from build123d import *

# Parameters (mm, degrees)
SKETCH1_W                           = 139.7
SKETCH1_H                           = 127
BOSS_EXTRUDE1_DEPTH                 = 12
F_8_CLEARANCE_HOLE1_D               = 4.9149
SKETCH2_R                           = 43.18
SKETCH2_R_2                         = 4.7625
CUT_EXTRUDE1_DEPTH                  = 1.27
SKETCH2_4_R                         = 4.7625
CUT_EXTRUDE2_DEPTH                  = 96.159195562
TAP_DRILL_FOR_10_24_TAP1_AT_2_COUNT = 2
TAP_DRILL_FOR_10_24_TAP1_AT_2_PITCH = 50.8
TAP_DRILL_FOR_10_24_TAP1_AT_3_COUNT = 2
TAP_DRILL_FOR_10_24_TAP1_AT_3_PITCH = 101.6
SKETCH8_R                           = 5.715
CUT_EXTRUDE3_DEPTH                  = 0.889


with BuildPart() as part:
    # Sketch1 → Boss-Extrude1 (new body)
    with BuildSketch(Plane(origin=(0, 0, 0), x_dir=(0, 0, -1), z_dir=(1, 0, 0))):
        Rectangle(SKETCH1_W, SKETCH1_H)
    extrude(amount=BOSS_EXTRUDE1_DEPTH)

    # #8 Clearance Hole1 (through all)
    with Locations(Plane.ZY):
        with Locations((-32.786915098, 34.756915098), (32.786915098, 34.756915098), (32.786915098, -30.816915098), (-32.786915098, -30.816915098)):
            Hole(F_8_CLEARANCE_HOLE1_D / 2)

    # Sketch2 → Cut-Extrude1 (cut)
    with BuildSketch(Plane.ZY):
        with Locations((0, 1.97)):
            Circle(SKETCH2_R)
        with Locations((0, 1.97)):
            Circle(SKETCH2_R_2, mode=Mode.SUBTRACT)
    extrude(amount=-CUT_EXTRUDE1_DEPTH, mode=Mode.SUBTRACT)

    # Sketch2<4> → Cut-Extrude2 (cut, through all)
    with BuildSketch(Plane.ZY):
        with Locations((0, 1.97)):
            Circle(SKETCH2_4_R)
    extrude(amount=-CUT_EXTRUDE2_DEPTH, mode=Mode.SUBTRACT)

    # Sketch7 → Tap Drill for #10-24 Tap1 (revolve, cut)
    with BuildSketch(Plane(origin=(6, -63.5, -50.8), x_dir=(0, 0, -1), z_dir=(1, 0, 0))):
        Polygon((0, 0), (0, 13.840824014), (1.89865, 12.7), (1.89865, 0), align=None)
    tap_drill_for_10_24_tap1 = revolve(axis=Axis((6, -69.85, -50.8), (0, 1, 0)), mode=Mode.SUBTRACT)

    # Tap Drill for #10-24 Tap1 at 2: Tap Drill for #10-24 Tap1 ×2
    with Locations(*[(0, 0, i * TAP_DRILL_FOR_10_24_TAP1_AT_2_PITCH) for i in range(1, TAP_DRILL_FOR_10_24_TAP1_AT_2_COUNT)]):
        add(tap_drill_for_10_24_tap1, mode=Mode.SUBTRACT)

    # Tap Drill for #10-24 Tap1 at 3: Tap Drill for #10-24 Tap1 ×2
    with Locations(*[(0, 0, i * TAP_DRILL_FOR_10_24_TAP1_AT_3_PITCH) for i in range(1, TAP_DRILL_FOR_10_24_TAP1_AT_3_COUNT)]):
        add(tap_drill_for_10_24_tap1, mode=Mode.SUBTRACT)

    # Mirror1: Tap Drill for #10-24 Tap1 across plane
    add(tap_drill_for_10_24_tap1.mirror(Plane.ZX), mode=Mode.SUBTRACT)

    # Mirror1 copy 1 sketch → Mirror1 copy 1 (revolve, cut)
    with BuildSketch(Plane(origin=(6, 63.5, 0), x_dir=(0, 0, -1), z_dir=(1, 0, 0))):
        Polygon((0, 0), (0, -13.840824014), (1.89865, -12.7), (1.89865, 0), align=None)
    revolve(axis=Axis((6, 69.85, 0), (0, 1, 0)), mode=Mode.SUBTRACT)

    # Mirror1 copy 2 sketch → Mirror1 copy 2 (revolve, cut)
    with BuildSketch(Plane(origin=(6, 63.5, 50.8), x_dir=(0, 0, -1), z_dir=(1, 0, 0))):
        Polygon((0, 0), (0, -13.840824014), (1.89865, -12.7), (1.89865, 0), align=None)
    revolve(axis=Axis((6, 69.85, 50.8), (0, 1, 0)), mode=Mode.SUBTRACT)

    # Sketch8 → Cut-Extrude3 (cut)
    with BuildSketch(Plane.ZY.offset(-1.27)):
        with Locations((0, 1.97)):
            Circle(SKETCH8_R)
    extrude(amount=-CUT_EXTRUDE3_DEPTH, mode=Mode.SUBTRACT)


solid = part.part
Can you work these out from the model? Positions are in its coordinate system, mm. A direction names the side the tool comes from. Give positions to 0.01 mm unless a question says otherwise; leave off trailing zeros. Loops run counter-clockwise (first coordinate to the right, second up) from the corner with the lowest first, then second, coordinate; pieces in that order, holes last. Notation, with made-up numbers: M 41.5,16 L 57.5,16 A30 ccw 57.5,41 Z; hole C -40,3 d5. An arc over 180 degrees is marked long. One line per item, written item: value. Start each with the question number.
1) I'm going to push flat-ended pins straight in: pin 1 (2.5 mm diameter, centred on x = 6, z = -50.8, fed in from +Y); pin 2 (3.5 mm diameter, centred on x = 6, z = 50.8, fed in from -Y); pin 3 (5.5 mm diameter, centred on y = 2.5, z = 2, fed in from -X). Where does each tip first touch, or does it pass through?
2) If we section it at B-B, the plane z = -19: Write out the boundary of the cut face in (x, y).
3) If I drill on line 1 (Z direction, x = 6, y = -58.25); line 2 (Y direction, x = 10.5, z = 32); line 3 (Z direction, x = 5.5, y = -56), over which ranges is the centre line in solid material (lowest first)? Write a range as [from, to].
4) If we section it at C-C, the plane y = 28.5: Write out the boundary of the cut face in (x, z).
5) If we section it at A-A, the plane y = -54: Write out the boundary of the cut face in (x, z), and give its area (3 significant figures).
6) On a 3-axis mill with a long thin cutter (end or side, diameter ignored), from which of +Z, -Z, +X, -X, +Y, -Y can I reach the whole of each face in a straight line? I mean faces 4 (the face through (7.155, 57.239, -49.293)), 5 (the face through (1.27, -7, -1)), 6 (the face through (6.08, -28.74, 31.47)), 7 (the face through (6.727, -57.239, -1.754)). Say none if no direction works.
7) Thinking about a two-plate mould opening in X: for faces 1 (the face through (4.4, 57.24, -1.02)), 2 (the face through (12, 15, 1)), 3 (the face through (6.084, 33.816, 30.517)), which applies, +X half, -X half, draft (parallel to the pull), parting line (faces both ways), or undercut?
Completed:
1. pin 1: stops at y = 50.41
1. pin 2: stops at y = -50.71
1. pin 3: stops at x = 2.16
2. outline: M 0,-63.5 L 12,-63.5 L 12,63.5 L 0,63.5 L 0,40.75 L 1.27,40.75 L 1.27,-36.81 L 0,-36.81 Z
3. line 1: z = [-69.85, -52.7], [-48.9, -1.9], [1.9, 48.9], [52.7, 69.85]
3. line 2: y = [-63.5, -33.14], [-28.49, 32.43], [37.08, 63.5]
3. line 3: z = [-69.85, -52.63], [-48.97, -1.83], [1.83, 48.97], [52.63, 69.85]
4. outline: M 0,-69.85 L 12,-69.85 L 12,69.85 L 0,69.85 L 0,34.07 L 1.27,34.07 L 1.27,-34.07 L 0,-34.07 Z
5. outline: M 0,-69.85 L 12,-69.85 L 12,69.85 L 0,69.85 Z; hole C 6,-50.8 d3.8; hole C 6,0 d3.8; hole C 6,50.8 d3.8
5. area: 1,640 mm^2
6. face 4: +Y
6. face 5: -X
6. face 6: +X, -X
6. face 7: -Y
7. face 1: undercut
7. face 2: +X half
7. face 3: draft
